```python
from build123d import *

# Parameters (mm, degrees)
BOSS_EXTRUDE1_DEPTH                = 6.35
SKETCH2_R                          = 5
CUT_EXTRUDE1_DEPTH                 = 7.35
F_6_CLEARANCE_HOLE1_D              = 3.7973
F_6_CLEARANCE_HOLE1_DEPTH          = 10
F_6_CLEARANCE_HOLE1_TIP            = 1.140824014
FILLET1_R                          = 4
F_10_CLEARANCE_HOLE1_D             = 5.1054
F_10_CLEARANCE_HOLE1_DEPTH         = 10
F_10_CLEARANCE_HOLE1_TIP           = 1.533816902
F_6_CLEARANCE_HOLE2_D              = 3.6576
TAP_DRILL_FOR_4_40_TAP1_AT_2_COUNT = 2
TAP_DRILL_FOR_4_40_TAP1_AT_2_PITCH = 12.7
TAP_DRILL_FOR_4_40_TAP1_AT_3_COUNT = 2
TAP_DRILL_FOR_4_40_TAP1_AT_3_PITCH = 87.179331478
TAP_DRILL_FOR_4_40_TAP1_AT_4_COUNT = 2
TAP_DRILL_FOR_4_40_TAP1_AT_4_PITCH = 99.516880161


with BuildPart() as part:
    # Sketch1 → Boss-Extrude1 (new body)
    with BuildSketch(Plane(origin=(0, 0, 0), x_dir=(1, 0, 0), z_dir=(0, 1, 0))):
        Polygon((-155, -27), (155, -27), (155, 27), (155, 62), (123, 62), (123, 27), (-123, 27), (-123, 62), (-155, 62), (-155, 27), align=None)
    extrude(amount=BOSS_EXTRUDE1_DEPTH)

    # Sketch2 → Cut-Extrude1 (cut, through all)
    with BuildSketch(Plane(origin=(0, 6.35, 0), x_dir=(1, 0, 0), z_dir=(0, 1, 0))):
        Circle(SKETCH2_R)
    extrude(amount=-CUT_EXTRUDE1_DEPTH, mode=Mode.SUBTRACT)

    # #6 Clearance Hole1
    with Locations(Plane(origin=(-145.915, 6.35, -54.265), x_dir=(0, 0, 1), z_dir=(0, 1, 0))):
        with Locations((0, 0), (0, 13.83), (13.83, 13.83), (13.83, 0), (6.915, 6.915), (52.35, 29), (52.35, 42.83), (66.18, 42.83), (66.18, 29), (59.265, 35.915), (32.265, 123.915), (32.265, 167.915), (76.265, 167.915), (76.265, 123.915), (66.18, 249), (52.35, 249), (52.35, 262.83), (66.18, 262.83), (59.265, 255.915), (13.83, 278), (6.915, 284.915), (0, 278), (0, 291.83), (13.83, 291.83)):
            Hole(F_6_CLEARANCE_HOLE1_D / 2, depth=F_6_CLEARANCE_HOLE1_DEPTH)
            with Locations((0, 0, -(F_6_CLEARANCE_HOLE1_DEPTH + F_6_CLEARANCE_HOLE1_TIP / 2))):  # 118° drill point
                Cone(0, F_6_CLEARANCE_HOLE1_D / 2, F_6_CLEARANCE_HOLE1_TIP, mode=Mode.SUBTRACT)

    # Fillet1
    fillet1_edges = [part.edges().sort_by_distance(p)[0] for p in [
        (155, 3.175, 27),
        (-155, 3.175, 27),
        (-155, 3.175, -62),
        (-123, 3.175, -62),
        (-123, 3.175, -27),
        (123, 3.175, -27),
        (123, 3.175, -62),
        (155, 3.175, -62),
    ]]
    fillet(fillet1_edges, radius=FILLET1_R)

    # #10 Clearance Hole1
    with Locations(Plane(origin=(-18.25, 6.35, 0), x_dir=(0, 0, 1), z_dir=(0, 1, 0))):
        with Locations((0, 0), (0, 36.5)):
            Hole(F_10_CLEARANCE_HOLE1_D / 2, depth=F_10_CLEARANCE_HOLE1_DEPTH)
            with Locations((0, 0, -(F_10_CLEARANCE_HOLE1_DEPTH + F_10_CLEARANCE_HOLE1_TIP / 2))):  # 118° drill point
                Cone(0, F_10_CLEARANCE_HOLE1_D / 2, F_10_CLEARANCE_HOLE1_TIP, mode=Mode.SUBTRACT)

    # #6 Clearance Hole2 (through all)
    with Locations(Plane(origin=(0, 6.35, 0), x_dir=(-1, 0, 0), z_dir=(0, 1, 0))):
        with Locations((90, -21.412), (90, 5.5374), (-90, 5.5374), (-90, -21.412), (80, -16.5352), (-80, -16.5352)):
            Hole(F_6_CLEARANCE_HOLE2_D / 2)

    # Sketch11 → Tap Drill for #4-40 Tap1 (revolve, cut)
    with BuildSketch(Plane(origin=(-150.684, 6.35, -28.7), x_dir=(0, 0, 1), z_dir=(1, 0, 0))):
        Polygon((0, 0), (0, 7.029152758), (1.1303, 6.35), (1.1303, 0), align=None)
    tap_drill_for_4_40_tap1 = revolve(axis=Axis((-150.684, 12.7, -28.7), (0, -1, 0)), mode=Mode.SUBTRACT)

    # Tap Drill for #4-40 Tap1 at 2: Tap Drill for #4-40 Tap1 ×2
    with Locations(*[(0, 0, i * TAP_DRILL_FOR_4_40_TAP1_AT_2_PITCH) for i in range(1, TAP_DRILL_FOR_4_40_TAP1_AT_2_COUNT)]):
        add(tap_drill_for_4_40_tap1, mode=Mode.SUBTRACT)

    # Tap Drill for #4-40 Tap1 at 3: Tap Drill for #4-40 Tap1 ×2
    with Locations(*[Vector(0.967362316, 0, 0.253397217) * (i * TAP_DRILL_FOR_4_40_TAP1_AT_3_PITCH) for i in range(1, TAP_DRILL_FOR_4_40_TAP1_AT_3_COUNT)]):
        add(tap_drill_for_4_40_tap1, mode=Mode.SUBTRACT)

    # Tap Drill for #4-40 Tap1 at 4: Tap Drill for #4-40 Tap1 ×2
    with Locations(*[Vector(0.975050663, 0, 0.221982441) * (i * TAP_DRILL_FOR_4_40_TAP1_AT_4_PITCH) for i in range(1, TAP_DRILL_FOR_4_40_TAP1_AT_4_COUNT)]):
        add(tap_drill_for_4_40_tap1, mode=Mode.SUBTRACT)

    # Mirror1: Tap Drill for #4-40 Tap1 across plane
    add(tap_drill_for_4_40_tap1.mirror(Plane(origin=(0, 0, 0), x_dir=(0, 0, 1), z_dir=(1, 0, 0))), mode=Mode.SUBTRACT)

    # Mirror1 copy 1 sketch → Mirror1 copy 1 (revolve, cut)
    with BuildSketch(Plane(origin=(150.684, 6.35, -16), x_dir=(0, 0, 1), z_dir=(-1, 0, 0))):
        Polygon((0, 0), (0, -7.029152758), (1.1303, -6.35), (1.1303, 0), align=None)
    revolve(axis=Axis((150.684, 12.7, -16), (0, 1, 0)), mode=Mode.SUBTRACT)

    # Mirror1 copy 2 sketch → Mirror1 copy 2 (revolve, cut)
    with BuildSketch(Plane(origin=(66.35, 6.35, -6.609), x_dir=(0, 0, 1), z_dir=(-1, 0, 0))):
        Polygon((0, 0), (0, -7.029152758), (1.1303, -6.35), (1.1303, 0), align=None)
    revolve(axis=Axis((66.35, 12.7, -6.609), (0, 1, 0)), mode=Mode.SUBTRACT)

    # Mirror1 copy 3 sketch → Mirror1 copy 3 (revolve, cut)
    with BuildSketch(Plane(origin=(53.65, 6.35, -6.609), x_dir=(0, 0, 1), z_dir=(-1, 0, 0))):
        Polygon((0, 0), (0, -7.029152758), (1.1303, -6.35), (1.1303, 0), align=None)
    revolve(axis=Axis((53.65, 12.7, -6.609), (0, 1, 0)), mode=Mode.SUBTRACT)


solid = part.part
```
Source: CAD feature listing. Evaluate the final solid. Frame: model axes, mm. A direction names the side the tool comes from. Coordinates: 2 decimals unless noted, no trailing zeros. Write each loop counter-clockwise with the first axis right and the second up, starting at its lowest first coordinate (ties: lowest second). Pieces come first, ordered by that corner, then holes. Notation, with made-up numbers: (46, -33.5) - (90, -33.5) arc R29 cw to (90, -9.5) - close; hole circle Ø6 at (40, 3). An arc over 180 degrees is marked (long way). Answer as a JSON object with one key per item and string values.
Q1. Section query B-B, the plane z = -34.5. Output: boundary loops of the cut face in (x, y), plus the area to 3 significant figures.
Ans:
{"outline": "(-155, 0) - (-123, 0) - (-123, 6.35) - (-155, 6.35) - close; (123, 0) - (155, 0) - (155, 6.35) - (123, 6.35) - close", "area": "406 mm2"}
Q2. Section query C-C, the plane y = 1.5. State how many separate pieces and enclosed holes the cut face has, plus the area to 3 significant figures.
Ans:
{"separate pieces": "1", "enclosed holes": "41", "area": "18,500 mm2"}
Q3. Material intervals for line 1 (X direction, y = 6.25, z = 12); line 2 (X direction, y = 4.5, z = -57); line 3 (X direction, y = 6.25, z = -7.5), sorted ascending. Write a range as [from, to].
Ans:
{"line 1": "x = [-155, -118.81], [-115.02, -104.98], [-101.19, 101.19], [104.98, 115.02], [118.81, 155]", "line 2": "x = [-155, -123], [123, 155]", "line 3": "x = [-155, -67.05], [-65.65, -54.35], [-52.95, 52.95], [54.35, 65.65], [67.05, 155]"}
Q4. Section query A-A, the plane x = 0. Output: boundary loops of the cut face in (y, z), plus the area to 3 significant figures.
Ans:
{"outline": "(0, -27) - (6.35, -27) - (6.35, -5) - (0, -5) - close; (0, 5) - (6.35, 5) - (6.35, 27) - (0, 27) - close", "area": "279 mm2"}
Q5. Set-up query: faces 5 (the cylindrical face through (-16.098, 3.131, -1.372)), 6 (the flat face through (123, 3, -45)). Return all of +Z, -Z, +X, -X, +Y, -Y with unobstructed straight access to the full face (end or side cutting, diameter ignored); none if empty.
Ans:
{"face 5": "+Y, -Y", "face 6": "-Z, +Y, -Y"}
Q6. Section query D-D, the plane x = -43. Output: boundary loops of the cut face in (y, z), plus the area to 3 significant figures.
Ans:
{"outline": "(0, -27) - (6.35, -27) - (6.35, 27) - (0, 27) - close", "area": "343 mm2"}
Q7. Draft query along Z for faces 1 (the flat face through (-123, 3, -44)), 2 (the cylindrical face through (-1.08, 3.22, 4.88)), 3 (the flat face through (139, 3, -62)), 4 (the flat face through (-2, 3, 27)). Return one class per face: released by +Z, released by -Z, zero draft, split by the parting line, or undercut.
Ans:
{"face 1": "zero draft", "face 2": "undercut", "face 3": "released by -Z", "face 4": "released by +Z"}
Q8. First-contact query: pin 1 Ø3.5 at (x, z) = (22, -22) entering from -Y; pin 2 Ø1.5 at (x, y) = (-115.5, 5) entering from -Z; pin 3 Ø3 at (x, y) = (-120, 2) entering from -Z. Flat tips, straight axial feed; report the tip coordinate or a pass-through.
Ans:
{"pin 1": "passes through", "pin 2": "stops at z = -27", "pin 3": "stops at z = -27.88"}
